CAD build for the part. Positions are in the model's coordinates, mm. A direction names the side the tool comes from. Coordinates: 2 decimals unless noted, no trailing zeros. Write each loop counter-clockwise with the first axis right and the second up, starting at its lowest first coordinate (ties: lowest second). Pieces come first, ordered by that corner, then holes. Notation, with made-up numbers: (-37.75, 83.5) - (-6.75, 83.5) arc R32 cw to (-6.75, 111.5) - close; hole circle Ø11 at (37.25, -32.75). An arc over 180 degrees is marked (long way). One line per question, with ' | ' between items. Start each with the question number.
1. Band-saw the part on C-C, the plane y = 28. Write the cut outline in (x, z), then the cut area to 3 significant figures.
2. Band-saw the part on B-B, the plane x = 19.5. Write the cut outline in (y, z).
3. Two-plate mould, pull along Z, no slides. Class faces 4 (the flat face through (20.162, 13.759, 2.465)), 5 (the flat face through (-10, -4, 95)), 6 (the flat face through (-7, 13.206, 85)): +Z half, -Z half, draft (parallel to the pull), parting line (faces both ways), or undercut.
4. Which spindle directions (+Z, -Z, +X, -X, +Y, -Y) get a long thin tool onto all of the face, cutting with end or side? Do faces 1 (the flat face through (-14, 26, 82.674)), 2 (the flat face through (0, 26, 74)), 3 (the flat face through (7.71, -34.544, 2.465)). Say none if no direction does.
5. Probe line 1 (Z direction, x = 6, y = 6); line 2 (Y direction, x = -19.5, z = 72); line 3 (X direction, y = -5, z = 13). List the from-to ranges inside material, lowest first.
6. Band-saw the part on D-D, the plane z = 62. Write the cut outline in (x, y).
7. Band-saw the part on A-A, the plane y = 11.5. Write the cut outline in (x, z), then the cut area to 3 significant figures.
8. Flat gauge pins, fed straight in: P1, Ø22.5, axis at y = -15, z = 36.5, coming from the +X side; P2, Ø20, axis at x = -9, y = 29.5, coming from the +Z side; P3, Ø6, axis at x = 3, z = 73.5, coming from the -Y side. Where does each tip first touch, or does it go through?
from build123d import *

# Parameters (mm, degrees)
F1_DEPTH = 50
F2_W     = 20
F2_H     = 20
F3_DEPTH = 10
F4_W     = 35
F4_H     = 35
F5_DEPTH = 35
F7_DEPTH = 5
F8_W     = 27.715054
F8_H     = 16.261809
F9_DEPTH = 25


with BuildPart() as f1:
    # F0 (on Top) → F1 (new body)
    with BuildSketch(Plane.XY):
        Polygon((-10.215054, 20.70647), (-35.215054, 20.70647), (-35.215054, -29.29353), (14.784946, -29.29353), (14.784946, 20.70647), (0, 20.70647), align=None)
    extrude(amount=F1_DEPTH)

    # F2 (on face) → F3 (join)
    with BuildSketch(Plane.XY.offset(50)):
        with Locations((-10.215054, -4.29353)):
            Rectangle(F2_W, F2_H)
    extrude(amount=F3_DEPTH)

    # F4 (on face) → F5 (join)
    with BuildSketch(Plane.XY.offset(60)):
        with Locations((-10.215054, -4.29353)):
            Rectangle(F4_W, F4_H)
    extrude(amount=F5_DEPTH)

    # F6 (on face) → F7 (join)
    with BuildSketch(Plane(origin=(0, 0, 0), x_dir=(1, 0, 0), z_dir=(0, 0, -1))):
        Polygon((-10.215054, 29.29353), (-45.821656, 39.900132), (-35.215054, 4.29353), (-45.570394, -31.061809), (-10.215054, -20.70647), (25.391547, -31.313071), (14.784946, 4.29353), (25.140285, 39.648869), align=None)
    extrude(amount=-F7_DEPTH)

    # F8 (on face) → F9 (join)
    with BuildSketch(Plane(origin=(0, 13.20647, 0), x_dir=(-1, 0, 0), z_dir=(0, 1, 0))):
        with Locations((13.857527, 74.543308)):
            Rectangle(F8_W, F8_H)
    extrude(amount=F9_DEPTH)


solid = f1.part
Filled in:
1) outline: (-44.67, 0) - (-35.12, 0) - (-35.12, 5) - (-44.67, 5) - close; (-27.72, 66.41) - (0, 66.41) - (0, 82.67) - (-27.72, 82.67) - close; (14.27, 0) - (24.4, 0) - (24.4, 5) - (14.27, 5) - close | area: 549 mm²
2) outline: (-38, 0) - (-20.39, 0) - (-20.39, 5) - (-38, 5) - close; (11.54, 0) - (29.56, 0) - (29.56, 5) - (11.54, 5) - close
3) face 4: draft | face 5: +Z half | face 6: undercut
4) face 1: +Z, +X, -X, +Y | face 2: +Z, +X, +Y | face 3: +Z, -Z, -Y
5) line 1: z = 0 to 50, 60 to 95 | line 2: y = -21.79 to 38.21 | line 3: x = -35.22 to 14.78
6) outline: (-27.72, -21.79) - (7.28, -21.79) - (7.28, 13.21) - (-27.72, 13.21) - close
7) outline: (-39.84, 0) - (19.49, 0) - (19.49, 5) - (14.78, 5) - (14.78, 50) - (-35.22, 50) - (-35.22, 5) - (-39.84, 5) - close; (-27.72, 60) - (7.28, 60) - (7.28, 95) - (-27.72, 95) - close | area: 3,770 mm²
8) P1: stops at x = 14.78 | P2: stops at z = 82.67 | P3: stops at y = -21.79
